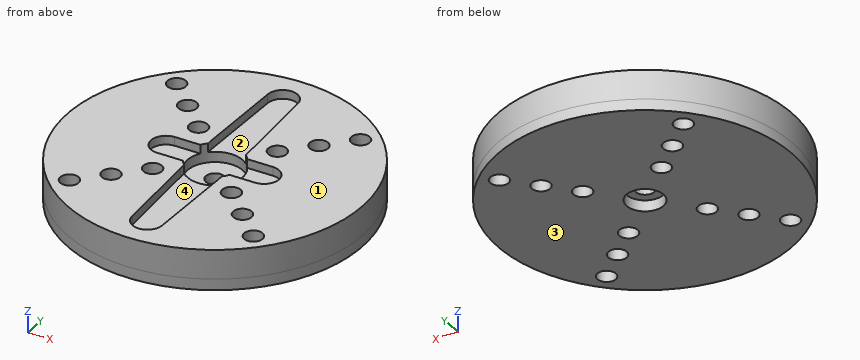
```python
from build123d import *

# Parameters (mm, degrees)
SKETCH1_R               = 20
BOSS_EXTRUDE1_DEPTH     = 4
SKETCH2_R               = 1.25
CUT_EXTRUDE1_DEPTH      = 29.565713714
CAVITY1_START           = 2.8
CAVITY1_OUTLINE_R       = 0.675
CAVITY1_OUTLINE_R_2     = 0.6
CAVITY1_OUTLINE_R_3     = 2.5
CAVITY1_DEPTH           = 1.2
CAVITY1_START_2         = 3.4
CAVITY1_2_OUTLINE_R     = 2.5
CAVITY1_2_OUTLINE_R_2   = 1.25
CAVITY1_2_DEPTH         = 0.6
CUT_EXTRUDE2_START      = -2
CUT_EXTRUDE2_DEPTH      = 2
CUT_EXTRUDE3_START      = -1.2
CUT_EXTRUDE3_DEPTH      = 1.2
CUT_EXTRUDE4_DEPTH      = 1.2
SKETCH6_R               = 1.25
CUT_EXTRUDE5_DEPTH      = 29.565713714
CIRPATTERN1_COUNT       = 4
CUT_EXTRUDE6_DEPTH      = 29.422526278
CUT_EXTRUDE6_DEPTH_BACK = 1.4
SKETCH7_R               = 3.75
SKETCH8_R               = 20
SKETCH8_R_2             = 2.5
SKETCH8_R_3             = 1.25
BOSS_EXTRUDE2_DEPTH     = 1.5


# Read off the part's stored shape, not the designer's step: Cavity1
with BuildPart() as part:
    # Sketch1 → Boss-Extrude1 (new body)
    with BuildSketch(Plane.XY):
        Circle(SKETCH1_R)
    extrude(amount=BOSS_EXTRUDE1_DEPTH)

    # Sketch2 → Cut-Extrude1 (cut, through all)
    with BuildSketch(Plane.XY.offset(4)):
        Circle(SKETCH2_R)
    extrude(amount=-CUT_EXTRUDE1_DEPTH, mode=Mode.SUBTRACT)

    # Cavity1 outline → Cavity1 (cut)
    with BuildSketch(Plane.XY.offset(CAVITY1_START)):
        with BuildLine():
            ThreePointArc((2.993325909, 2), (2.762479071, 2.308399745), (2.5, 2.590366769))
            Line((2.5, 2.590366769), (2.5, 3.6))
            Line((2.5, 3.6), (2, 15.6))
            ThreePointArc((2, 15.6), (0, 17.6), (-2, 15.6))
            Line((-2, 15.6), (-2.5, 3.6))
            Line((-2.5, 3.6), (-2.5, 2.590366769))
            ThreePointArc((-2.5, 2.590366769), (-2.762479071, 2.308399745), (-2.993325909, 2))
            Line((-2.993325909, 2), (-6.6, 2))
            ThreePointArc((-6.6, 2), (-8.6, 0), (-6.6, -2))
            Line((-6.6, -2), (-2.993325909, -2))
            ThreePointArc((-2.993325909, -2), (-2.762479071, -2.308399745), (-2.5, -2.590366769))
            Line((-2.5, -2.590366769), (-2.5, -3.6))
            Line((-2.5, -3.6), (-2, -15.6))
            ThreePointArc((-2, -15.6), (0, -17.6), (2, -15.6))
            Line((2, -15.6), (2.5, -3.6))
            Line((2.5, -3.6), (2.5, -2.590366769))
            ThreePointArc((2.5, -2.590366769), (2.762479071, -2.308399745), (2.993325909, -2))
            Line((2.993325909, -2), (6.6, -2))
            ThreePointArc((6.6, -2), (8.6, 0), (6.6, 2))
            Line((6.6, 2), (2.993325909, 2))
        make_face()
        with Locations((0, -15.6)):
            Circle(CAVITY1_OUTLINE_R, mode=Mode.SUBTRACT)
        with Locations((0, -13.4)):
            Circle(CAVITY1_OUTLINE_R, mode=Mode.SUBTRACT)
        with Locations((0, -11.2)):
            Circle(CAVITY1_OUTLINE_R, mode=Mode.SUBTRACT)
        with Locations((0, -9)):
            Circle(CAVITY1_OUTLINE_R, mode=Mode.SUBTRACT)
        with Locations((0, -6.8)):
            Circle(CAVITY1_OUTLINE_R, mode=Mode.SUBTRACT)
        with Locations((0, -4.6)):
            Circle(CAVITY1_OUTLINE_R, mode=Mode.SUBTRACT)
        with Locations((-6.6, 0)):
            Circle(CAVITY1_OUTLINE_R_2, mode=Mode.SUBTRACT)
        with Locations((-4.6, 0)):
            Circle(CAVITY1_OUTLINE_R_2, mode=Mode.SUBTRACT)
        Circle(CAVITY1_OUTLINE_R_3, mode=Mode.SUBTRACT)
        with Locations((0, 4.6)):
            Circle(CAVITY1_OUTLINE_R, mode=Mode.SUBTRACT)
        with Locations((0, 6.8)):
            Circle(CAVITY1_OUTLINE_R, mode=Mode.SUBTRACT)
        with Locations((4.6, 0)):
            Circle(CAVITY1_OUTLINE_R_2, mode=Mode.SUBTRACT)
        with Locations((6.6, 0)):
            Circle(CAVITY1_OUTLINE_R_2, mode=Mode.SUBTRACT)
        with Locations((0, 9)):
            Circle(CAVITY1_OUTLINE_R, mode=Mode.SUBTRACT)
        with Locations((0, 11.2)):
            Circle(CAVITY1_OUTLINE_R, mode=Mode.SUBTRACT)
        with Locations((0, 13.4)):
            Circle(CAVITY1_OUTLINE_R, mode=Mode.SUBTRACT)
        with Locations((0, 15.6)):
            Circle(CAVITY1_OUTLINE_R, mode=Mode.SUBTRACT)
    extrude(amount=CAVITY1_DEPTH, mode=Mode.SUBTRACT)

    # Cavity1 2 outline → Cavity1 2 (cut)
    with BuildSketch(Plane.XY.offset(CAVITY1_START_2)):
        Circle(CAVITY1_2_OUTLINE_R)
        Circle(CAVITY1_2_OUTLINE_R_2, mode=Mode.SUBTRACT)
    extrude(amount=CAVITY1_2_DEPTH, mode=Mode.SUBTRACT)

    # Sketch3 → Cut-Extrude2 (cut)
    with BuildSketch(Plane.XY.offset(3.4).offset(CUT_EXTRUDE2_START)):
        with BuildLine():
            ThreePointArc((-2.5, 0), (0, -2.5), (2.5, 0))
            ThreePointArc((2.5, 0), (0, 2.5), (-2.5, 0))
        make_face()
    extrude(amount=CUT_EXTRUDE2_DEPTH, mode=Mode.SUBTRACT)

    # Sketch4 → Cut-Extrude3 (cut)
    with BuildSketch(Plane.XY.offset(4).offset(CUT_EXTRUDE3_START)):
        with BuildLine():
            Line((-6.6, -2), (-2.993325909, -2))
            ThreePointArc((-2.993325909, -2), (-2.762479071, -2.308399745), (-2.5, -2.590366769))
            Line((-2.5, -2.590366769), (-2.5, -3.6))
            Line((-2.5, -3.6), (-2, -15.6))
            ThreePointArc((-2, -15.6), (0, -17.6), (2, -15.6))
            Line((2, -15.6), (2.5, -3.6))
            Line((2.5, -3.6), (2.5, -2.590366769))
            ThreePointArc((2.5, -2.590366769), (2.762479071, -2.308399745), (2.993325909, -2))
            Line((2.993325909, -2), (6.6, -2))
            ThreePointArc((6.6, -2), (8.6, 0), (6.6, 2))
            Line((6.6, 2), (2.993325909, 2))
            ThreePointArc((2.993325909, 2), (2.762479071, 2.308399745), (2.5, 2.590366769))
            Line((2.5, 2.590366769), (2.5, 3.6))
            Line((2.5, 3.6), (2, 15.6))
            ThreePointArc((2, 15.6), (0, 17.6), (-2, 15.6))
            Line((-2, 15.6), (-2.5, 3.6))
            Line((-2.5, 3.6), (-2.5, 2.590366769))
            ThreePointArc((-2.5, 2.590366769), (-2.762479071, 2.308399745), (-2.993325909, 2))
            Line((-2.993325909, 2), (-6.6, 2))
            ThreePointArc((-6.6, 2), (-8.6, 0), (-6.6, -2))
        make_face()
    extrude(amount=CUT_EXTRUDE3_DEPTH, mode=Mode.SUBTRACT)

    # Sketch5 → Cut-Extrude4 (cut)
    with BuildSketch(Plane.XY.offset(4)):
        with BuildLine():
            Line((-6.6, -2.03), (-3.00931886, -2.03))
            ThreePointArc((-3.00931886, -2.03), (-2.784441978, -2.328901645), (-2.53, -2.603075105))
            Line((-2.53, -2.603075105), (-2.53, -3.600624729))
            Line((-2.53, -3.600624729), (-2.029999903, -15.600627053))
            ThreePointArc((-2.029999903, -15.600627053), (0, -17.63), (2.029999903, -15.600627053))
            Line((2.029999903, -15.600627053), (2.53, -3.600624729))
            Line((2.53, -3.600624729), (2.53, -2.603075105))
            ThreePointArc((2.53, -2.603075105), (2.784441978, -2.328901645), (3.00931886, -2.03))
            Line((3.00931886, -2.03), (6.6, -2.03))
            ThreePointArc((6.6, -2.03), (8.63, 0), (6.6, 2.03))
            Line((6.6, 2.03), (3.00931886, 2.03))
            ThreePointArc((3.00931886, 2.03), (2.784441978, 2.328901645), (2.53, 2.603075105))
            Line((2.53, 2.603075105), (2.53, 3.600624729))
            Line((2.53, 3.600624729), (2.029999903, 15.600627053))
            ThreePointArc((2.029999903, 15.600627053), (0, 17.63), (-2.029999903, 15.600627053))
            Line((-2.029999903, 15.600627053), (-2.53, 3.600624729))
            Line((-2.53, 3.600624729), (-2.53, 2.603075105))
            ThreePointArc((-2.53, 2.603075105), (-2.784441978, 2.328901645), (-3.00931886, 2.03))
            Line((-3.00931886, 2.03), (-6.6, 2.03))
            ThreePointArc((-6.6, 2.03), (-8.63, 0), (-6.6, -2.03))
        make_face()
    extrude(amount=-CUT_EXTRUDE4_DEPTH, mode=Mode.SUBTRACT)

    # Sketch6 → Cut-Extrude5 (cut, through all)
    with BuildSketch(Plane.XY.offset(4)):
        with Locations((5.303300859, 5.303300859)):
            Circle(SKETCH6_R)
        with Locations((8.838834765, 8.838834765)):
            Circle(SKETCH6_R)
        with Locations((12.374368671, 12.374368671)):
            Circle(SKETCH6_R)
    cut_extrude5 = extrude(amount=-CUT_EXTRUDE5_DEPTH, mode=Mode.SUBTRACT)

    # CirPattern1: Cut-Extrude5 ×4 about axis
    cirpattern1_axis = Axis((0, 0, 0), (0, 0, 1))
    for i in range(1, CIRPATTERN1_COUNT):
        add(cut_extrude5.rotate(cirpattern1_axis, i * 360 / CIRPATTERN1_COUNT), mode=Mode.SUBTRACT)

    # Sketch7 → Cut-Extrude6 (cut, two sides: drawn at the far end of the back side and taken through both)
    with BuildSketch(Plane.XY.offset(2.8).offset(-CUT_EXTRUDE6_DEPTH_BACK)):
        with Locations(Location((0, 0, 0), (0, 0, 147.225549173))):
            Circle(SKETCH7_R)
    extrude(amount=CUT_EXTRUDE6_DEPTH + CUT_EXTRUDE6_DEPTH_BACK, mode=Mode.SUBTRACT)

    # Sketch8 → Boss-Extrude2 (add)
    with BuildSketch(Plane(origin=(0, 0, 0), x_dir=(-1, 0, 0), z_dir=(0, 0, -1))):
        Circle(SKETCH8_R)
        Circle(SKETCH8_R_2, mode=Mode.SUBTRACT)
        with Locations(Location((12.374368671, 12.374368671, 0), (0, 0, 90))):
            Circle(SKETCH8_R_3, mode=Mode.SUBTRACT)
        with Locations(Location((-12.374368671, 12.374368671, 0), (0, 0, 180))):
            Circle(SKETCH8_R_3, mode=Mode.SUBTRACT)
        with Locations(Location((-8.838834765, 8.838834765, 0), (0, 0, 180))):
            Circle(SKETCH8_R_3, mode=Mode.SUBTRACT)
        with Locations(Location((-5.303300859, 5.303300859, 0), (0, 0, 180))):
            Circle(SKETCH8_R_3, mode=Mode.SUBTRACT)
        with Locations((12.374368671, -12.374368671)):
            Circle(SKETCH8_R_3, mode=Mode.SUBTRACT)
        with Locations((8.838834765, -8.838834765)):
            Circle(SKETCH8_R_3, mode=Mode.SUBTRACT)
        with Locations((5.303300859, -5.303300859)):
            Circle(SKETCH8_R_3, mode=Mode.SUBTRACT)
        with Locations(Location((-12.374368671, -12.374368671, 0), (0, 0, 270))):
            Circle(SKETCH8_R_3, mode=Mode.SUBTRACT)
        with Locations(Location((-8.838834765, -8.838834765, 0), (0, 0, 270))):
            Circle(SKETCH8_R_3, mode=Mode.SUBTRACT)
        with Locations(Location((-5.303300859, -5.303300859, 0), (0, 0, 270))):
            Circle(SKETCH8_R_3, mode=Mode.SUBTRACT)
        with Locations(Location((5.303300859, 5.303300859, 0), (0, 0, 90))):
            Circle(SKETCH8_R_3, mode=Mode.SUBTRACT)
        with Locations(Location((8.838834765, 8.838834765, 0), (0, 0, 90))):
            Circle(SKETCH8_R_3, mode=Mode.SUBTRACT)
    extrude(amount=BOSS_EXTRUDE2_DEPTH)


solid = part.part
```
Geometry check sheet. Reference: the model listing, model coordinates, mm. Face numbers are marked on the shaded views. A direction names the side the tool comes from. Round coordinates to 2 decimals unless told otherwise and drop trailing zeros. Loops run counter-clockwise (first coordinate to the right, second up) from the corner with the lowest first, then second, coordinate; pieces in that order, holes last. Notation, with made-up numbers: (68, 6) - (123, 6) arc R21 cw to (123, 34) - close; hole circle Ø1 at (31.5, 77). An arc over 180 degrees is marked (long way). Use a Markdown table: item, result.
Q1. Cross-section at B-B on x = 0. Record the cut outline in (y, z).
Solutions:
| item | result |
|---|---|
| outline | (-20, -1.5) - (-2.5, -1.5) - (-2.5, 0) - (-1.25, 0) - (-1.25, 1.4) - (-3.75, 1.4) - (-3.75, 2.8) - (-17.63, 2.8) - (-17.63, 4) - (-20, 4) - close; (1.25, 0) - (2.5, 0) - (2.5, -1.5) - (20, -1.5) - (20, 4) - (17.63, 4) - (17.63, 2.8) - (3.75, 2.8) - (3.75, 1.4) - (1.25, 1.4) - close |
Q2. Draft check along X on the marked faces 3 and 4. Enter one of: released by +X, released by -X, zero draft, split by the parting line, or undercut.
Solutions:
| item | result |
|---|---|
| face 3 | zero draft |
| face 4 | undercut |
Q3. Access from +Z, -Z, +X, -X, +Y, -Y to the whole of each face (thin tool, end or side, straight path). Record for the marked faces 1 and 2.
Solutions:
| item | result |
|---|---|
| face 1 | +Z, +X, -X, +Y, -Y |
| face 2 | +Z |
Q4. Cross-section at C-C on z = -1. State how many separate pieces and enclosed holes the cut face has, plus the area to 3 significant figures.
Solutions:
| item | result |
|---|---|
| separate pieces | 1 |
| enclosed holes | 13 |
| area | 1,180 mm2 |
Q5. Cross-section at A-A on y = 0. Record the cut outline in (x, z).
Solutions:
| item | result |
|---|---|
| outline | (-20, -1.5) - (-2.5, -1.5) - (-2.5, 0) - (-1.25, 0) - (-1.25, 1.4) - (-3.75, 1.4) - (-3.75, 2.8) - (-8.63, 2.8) - (-8.63, 4) - (-20, 4) - close; (1.25, 0) - (2.5, 0) - (2.5, -1.5) - (20, -1.5) - (20, 4) - (8.63, 4) - (8.63, 2.8) - (3.75, 2.8) - (3.75, 1.4) - (1.25, 1.4) - close |
Q6. Material ranges on line 1 (X direction, y = 13, z = 2.6); line 2 (Y direction, x = 12, z = 3); line 3 (X direction, y = -12, z = 3.15), recorded low to high.
Solutions:
| item | result |
|---|---|
| line 1 | x = -15.2 to -13.46, -11.29 to 11.29, 13.46 to 15.2 |
| line 2 | y = -16 to -13.57, -11.18 to 11.18, 13.57 to 16 |
| line 3 | x = -16 to -13.57, -11.18 to -2.18, 2.18 to 11.18, 13.57 to 16 |
Q7. Go/stop test with flat-tipped pins: P1, Ø2, axis at x = 14.5, z = -1, coming from the +Y side; P2, Ø1.5, axis at x = 0, y = 11, coming from the +Z side; P3, Ø2, axis at x = -13, z = 2, coming from the -Y side. Record where each tip stops, or that it passes through.
Solutions:
| item | result |
|---|---|
| P1 | stops at y = 14.76 |
| P2 | stops at z = 2.8 |
| P3 | stops at y = -16 |
Q8. Cross-section at D-D on y = -9.5. Record the cut outline in (x, z).
Solutions:
| item | result |
|---|---|
| outline | (-17.6, -1.5) - (-9.9, -1.5) - (-9.9, 4) - (-17.6, 4) - close; (-7.78, -1.5) - (7.78, -1.5) - (7.78, 4) - (2.28, 4) - (2.28, 2.8) - (-2.28, 2.8) - (-2.28, 4) - (-7.78, 4) - close; (9.9, -1.5) - (17.6, -1.5) - (17.6, 4) - (9.9, 4) - close |
